from build123d import *

# Parameters (mm, degrees)
SKETCH1_W           = 30
SKETCH1_H           = 3
SKETCH1_W_2         = 3
SKETCH1_H_2         = 30
BOSS_EXTRUDE1_DEPTH = 3


with BuildPart() as part:
    # Sketch1 → Boss-Extrude1 (new body)
    with BuildSketch(Plane(origin=(0, 0, 0), x_dir=(1, 0, 0), z_dir=(0, 1, 0))):
        with Locations((0, -56)):
            Rectangle(SKETCH1_W, SKETCH1_H)
        with Locations((-56, 0)):
            Rectangle(SKETCH1_W_2, SKETCH1_H_2)
        with Locations((0, 56)):
            Rectangle(SKETCH1_W, SKETCH1_H)
        Polygon((-54.5, -54.5), (-54.5, -15), (-54.5, 15), (-54.5, 54.5), (-15, 54.5), (15, 54.5), (54.5, 54.5), (54.5, 15), (54.5, -15), (54.5, -54.5), (15, -54.5), (-15, -54.5), align=None)
        with Locations((56, 0)):
            Rectangle(SKETCH1_W_2, SKETCH1_H_2)
    extrude(amount=BOSS_EXTRUDE1_DEPTH)


solid = part.part
Read the model definition and answer for the solid it produces. Units are mm, in the model's axes. A direction names the side the tool comes from. Coordinates: 2 decimals unless noted, no trailing zeros. Order: outer loops, then holes, each group sorted by start corner. A loop starts at its lowest first (then second) coordinate and runs counter-clockwise, first axis right, second up. Notation, with made-up numbers: (57, 39) -> (63, 39) arc R18 ccw to (63, 71) -> close; hole circle Ø9 at (-10.5, -39.5). An arc over 180 degrees is marked (long way). Answer as a JSON object with one key per item and string values.
1) Each of these flat-tipped pins is pushed along its axis until it touches: pin 1 (1.5 mm diameter, centred on x = -55.5, y = 1.5, fed in from +Z); pin 2 (1.5 mm diameter, centred on y = 2, z = 55.5, fed in from +X); pin 3 (1.5 mm diameter, centred on x = -55.5, y = 2, fed in from -Z). Where does it stop, or does it pass through?
Model answer:
{"pin 1": "stops at z = 15", "pin 2": "stops at x = 15", "pin 3": "stops at z = -15"}
2) A cutting plane is placed at A-A, the plane y = 2.25. Determine the outline of the cut face in (x, z), plus the area to 3 significant figures.
Model answer:
{"outline": "(-57.5, -15) -> (-54.5, -15) -> (-54.5, -54.5) -> (-15, -54.5) -> (-15, -57.5) -> (15, -57.5) -> (15, -54.5) -> (54.5, -54.5) -> (54.5, -15) -> (57.5, -15) -> (57.5, 15) -> (54.5, 15) -> (54.5, 54.5) -> (15, 54.5) -> (15, 57.5) -> (-15, 57.5) -> (-15, 54.5) -> (-54.5, 54.5) -> (-54.5, 15) -> (-57.5, 15) -> close", "area": "12,200 mm²"}
3) Consider line 1 along X through (y, z) = (0.35, 24.5). Determine where the line is inside the solid, lowest interval first. Write a range as from..to.
Model answer:
{"line 1": "x = -54.5..54.5"}
4) A cutting plane is placed at C-C, the plane x = 19. Determine the outline of the cut face in (y, z), plus the area to 3 significant figures.
Model answer:
{"outline": "(0, -54.5) -> (3, -54.5) -> (3, 54.5) -> (0, 54.5) -> close", "area": "327 mm²"}
5) A cutting plane is placed at B-B, the plane z = 45.5. Determine the outline of the cut face in (x, y), plus the area to 3 significant figures.
Model answer:
{"outline": "(-54.5, 0) -> (54.5, 0) -> (54.5, 3) -> (-54.5, 3) -> close", "area": "327 mm²"}
6) A tool of negligible diameter and unlimited length cuts with its end or side. For faces 1 (the face through (34, 1, -54.5)), 2 (the face through (-15, 1, -56)), 3 (the face through (0, 1, -57.5)), 4 (the face through (-56, 1, 15)), 5 (the face through (54.5, 1, 35)), from which of +Z, -Z, +X, -X, +Y, -Y can it reach the whole face along a straight path? Write none if from no direction.
Model answer:
{"face 1": "-Z, +X, +Y, -Y", "face 2": "-Z, -X, +Y, -Y", "face 3": "-Z, +X, -X, +Y, -Y", "face 4": "+Z, -X, +Y, -Y", "face 5": "+Z, +X, +Y, -Y"}
